Job drawing, mm, ordinate dimensions from the low corner. One solid piece. Give positions to 0.01 mm unless a question says otherwise; leave off trailing zeros. Order: outer loops, then holes, each group sorted by start corner. A loop starts at its lowest first (then second) coordinate and runs counter-clockwise, first axis right, second up. Notation, with made-up numbers: (20.25, 42.5) - (44.25, 42.5) arc R33 cw to (44.25, 70.5) - close; hole circle Ø6 at (80, -29). An arc over 180 degrees is marked (long way). Write each question's results on one line, items separated by ' | '. Start each with the question number.
1) Cut at B-B on x = 3.4. List the corners of the cut face in (y, z) (1 decimal).
2) Drop flat-ended pins along their axis: pin 1 Ø1 at (x, y) = (3.5, 146) entering from -Z; pin 2 Ø1.5 at (x, z) = (2, 54) entering from -Y. Give the stop position or say it passes through.
3) Cut at D-D on z = 51.5. List the corners of the cut face in (x, y) (1 decimal).
4) Drill centre lines: line 1 along Z through (x, y) = (0.7, 16) (1 decimal); line 2 along Z through (x, y) = (3.1, 309) (1 decimal); line 3 along Z through (x, y) = (1.1, 155.5). Where is each one in solid material? Low to high. Write a range as from..to.
5) Cut at A-A on z = 10. List the corners of the cut face in (x, y), plus the area to 3 significant figures.
6) Cut at C-C on y = 43.5. List the corners of the cut face in (x, z) (1 decimal).
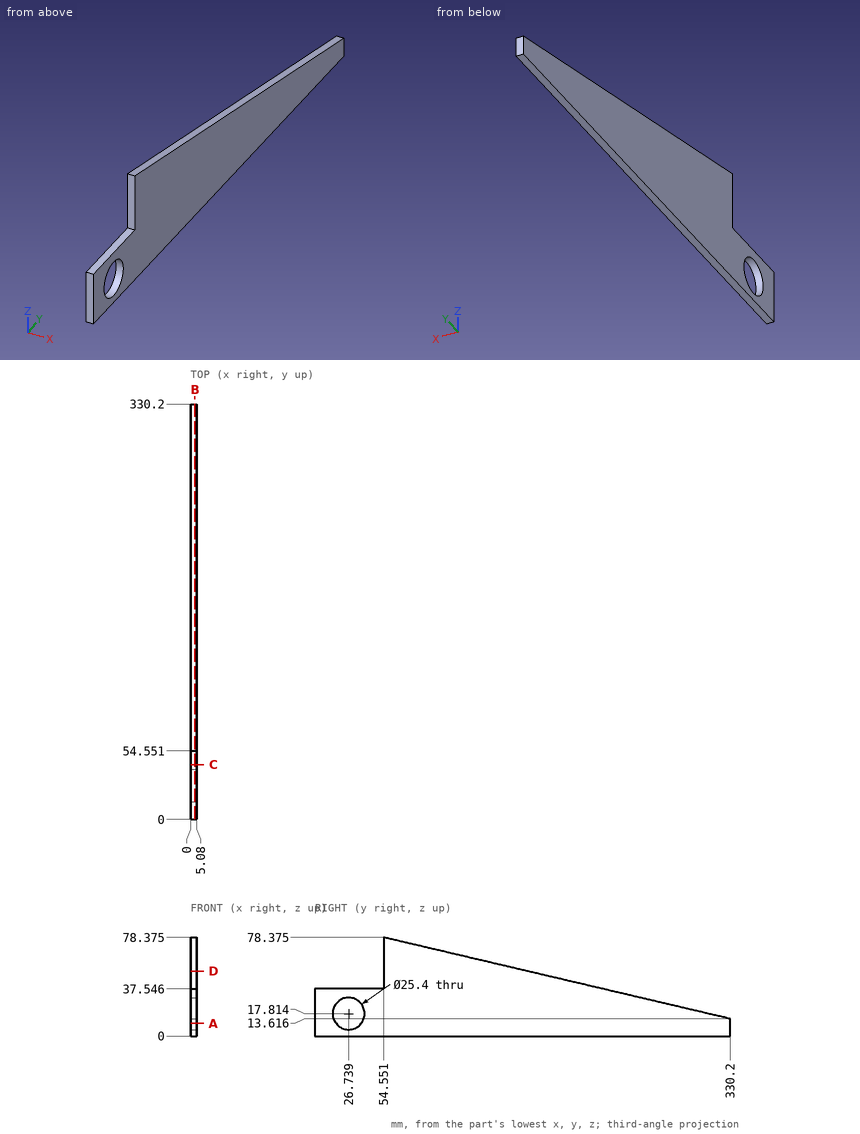
Results:
1) outline: (0, 0) - (330.2, 0) - (330.2, 13.6) - (54.6, 78.4) - (54.6, 37.5) - (0, 37.5) - close; hole circle Ø25.4 at (26.7, 17.8)
2) pin 1: z = 0 | pin 2: y = 54.55
3) outline: (0, 54.6) - (5.1, 54.6) - (5.1, 168.9) - (0, 168.9) - close
4) line 1: 0..11, 24.6..37.5 | line 2: 0..18.6 | line 3: 0..54.66
5) outline: (0, 0) - (5.08, 0) - (5.08, 16.73) - (0, 16.73) - close; (0, 36.75) - (5.08, 36.75) - (5.08, 330.2) - (0, 330.2) - close | area: 1,580 mm^2
6) outline: (0, 0) - (5.1, 0) - (5.1, 37.5) - (0, 37.5) - close
